from build123d import *

# Parameters (mm, degrees)
SKETCH1_R                      = 20.32
CYLINDER_DEPTH                 = 26.162
SKETCH18_R                     = 12.7
CUT_EXTRUDE10_DEPTH            = 23.368
SKETCH19_R                     = 1.905
CUT_EXTRUDE12_REACH            = 40.862
SKETCH21_R                     = 1.27
CIRPATTERN4_COUNT              = 6
CUT_EXTRUDE13_REACH            = 39.039
SKETCH22_R                     = 8.001
CUT_EXTRUDE15_REACH            = 54.431
CUT_EXTRUDE15_END_MAJOR_RADIUS = 12.573
CUT_EXTRUDE15_END_MINOR_RADIUS = 1.905
SKETCH25_R                     = 1.905
CIRPATTERN6_COUNT              = 2
SKETCH26_R                     = 1.905
CUT_EXTRUDE16_DEPTH            = 53.430547027
CUT_EXTRUDE17_DEPTH            = 39.862000188
CUT_EXTRUDE17_DEPTH_BACK       = 39.862000188
SKETCH27_W                     = 40.64
SKETCH27_H                     = 2.54


with BuildPart() as part:
    # Sketch1 → Cylinder (new body)
    with BuildSketch(Plane(origin=(0, 0, 0), x_dir=(1, 0, 0), z_dir=(0, 1, 0))):
        with Locations(Location((0, 0, 0), (0, 0, 270))):
            Circle(SKETCH1_R)
    extrude(amount=CYLINDER_DEPTH)

    # Sketch18 → Cut-Extrude10 (cut)
    with BuildSketch(Plane(origin=(0, 26.162, 0), x_dir=(1, 0, 0), z_dir=(0, 1, 0))):
        with Locations(Location((0, 0, 0), (0, 0, 270))):
            Circle(SKETCH18_R)
    extrude(amount=-CUT_EXTRUDE10_DEPTH, mode=Mode.SUBTRACT)

    # Sketch19 → Cut-Revolve7 (revolve, cut)
    with BuildSketch(Plane.XY, mode=Mode.PRIVATE) as cut_revolve7_sk:
        with Locations((12.573, 0)):
            Circle(SKETCH19_R)
    revolve(cut_revolve7_sk.sketch.rotate(Axis((0, 13.335, 0), (0, -1, 0)), 90), axis=Axis((0, 13.335, 0), (0, -1, 0)), mode=Mode.SUBTRACT)

    # Sketch21 → Cut-Extrude12 (cut, up to next)
    with BuildSketch(Plane(origin=(0, 26.162, 0), x_dir=(1, 0, 0), z_dir=(0, 1, 0)), mode=Mode.PRIVATE) as cut_extrude12_sk1:
        with Locations(Location((0, 17.78, 0), (0, 0, 270))):
            Circle(SKETCH21_R)
    cut_extrude12_tool1 = extrude(cut_extrude12_sk1.sketch, amount=-CUT_EXTRUDE12_REACH, mode=Mode.PRIVATE) & part.part
    cut_extrude12 = cut_extrude12_tool1.solids().sort_by_distance((0, 26.162, -17.78))[0]
    add(cut_extrude12, mode=Mode.SUBTRACT)

    # CirPattern4: Cut-Extrude12 ×6 about axis
    cirpattern4_axis = Axis((0, 0, 0), (0, 1, 0))
    for i in range(1, CIRPATTERN4_COUNT):
        add(cut_extrude12.rotate(cirpattern4_axis, i * 360 / CIRPATTERN4_COUNT), mode=Mode.SUBTRACT)

    # Sketch22 → Cut-Extrude13 (cut, up to next)
    with BuildSketch(Plane(origin=(0, 2.794, 0), x_dir=(1, 0, 0), z_dir=(0, 1, 0)), mode=Mode.PRIVATE) as cut_extrude13_sk1:
        with Locations(Location((0, 0, 0), (0, 0, 270))):
            Circle(SKETCH22_R)
    cut_extrude13_tool1 = extrude(cut_extrude13_sk1.sketch, amount=-CUT_EXTRUDE13_REACH, mode=Mode.PRIVATE) & part.part
    add(cut_extrude13_tool1.solids().sort_by_distance((0, 2.794, 0))[0], mode=Mode.SUBTRACT)

    # Cut-Extrude15: up to this torus (the profile starts outside it)
    cut_extrude15_end = Plane(origin=(0, 0, 0), z_dir=(0, 1, 0)) * Torus(CUT_EXTRUDE15_END_MAJOR_RADIUS, CUT_EXTRUDE15_END_MINOR_RADIUS, mode=Mode.PRIVATE)
    # Sketch25 → Cut-Extrude15 (cut, up to the surface)
    with BuildSketch(Plane(origin=(20.32, 0, 0), x_dir=(0, 0, -1), z_dir=(1, 0, 0)), mode=Mode.PRIVATE) as cut_extrude15_sk1:
        Circle(SKETCH25_R)
    cut_extrude15_tool1 = extrude(cut_extrude15_sk1.sketch, amount=-CUT_EXTRUDE15_REACH, mode=Mode.PRIVATE) - cut_extrude15_end
    cut_extrude15 = cut_extrude15_tool1.solids().sort_by_distance((20.32, 0, 0))[0]
    add(cut_extrude15, mode=Mode.SUBTRACT)

    # CirPattern6: Cut-Extrude15 ×2 about axis
    cirpattern6_axis = Axis((0, 13.335, 0), (0, -1, 0))
    for i in range(1, CIRPATTERN6_COUNT):
        add(cut_extrude15.rotate(cirpattern6_axis, i * 360 / CIRPATTERN6_COUNT), mode=Mode.SUBTRACT)

    # Sketch26 → Cut-Extrude16 (cut, through all)
    with BuildSketch(Plane(origin=(20.32, 0, 0), x_dir=(0, 0, -1), z_dir=(1, 0, 0))):
        with Locations((0, 10.922)):
            Circle(SKETCH26_R)
    extrude(amount=-CUT_EXTRUDE16_DEPTH, mode=Mode.SUBTRACT)

    # Sketch27 → Cut-Extrude17 (cut, two sides: drawn at the far end of the back side and taken through both)
    with BuildSketch(Plane.XY.offset(-CUT_EXTRUDE17_DEPTH_BACK)):
        with Locations((0, 24.892)):
            Rectangle(SKETCH27_W, SKETCH27_H)
    extrude(amount=CUT_EXTRUDE17_DEPTH + CUT_EXTRUDE17_DEPTH_BACK, mode=Mode.SUBTRACT)


solid = part.part
Source: CAD feature listing. Evaluate the final solid. Frame: model axes, mm. A direction names the side the tool comes from. Round coordinates to 2 decimals unless told otherwise and drop trailing zeros. Order: outer loops, then holes, each group sorted by start corner. A loop starts at its lowest first (then second) coordinate and runs counter-clockwise, first axis right, second up. Notation, with made-up numbers: (49, 4.5) - (89, 4.5) arc R22 cw to (89, 29.5) - close; hole circle Ø9 at (-23.5, 15). An arc over 180 degrees is marked (long way). Use a Markdown table: item, result. Add a question column.
1. Section query C-C (y = 11.5). Return the cut outline in (x, z) (3 decimals), then the cut area to 3 significant figures.
2. First-contact query: pin 1 (10 mm diameter, centred on y = 2.5, z = -13, fed in from +X); pin 2 (2.5 mm diameter, centred on y = 10.922, z = 0, fed in from -X); pin 3 (3 mm diameter, centred on x = -16, y = 7, fed in from +Z); pin 4 (1.5 mm diameter, centred on x = 7, y = 6.5, fed in from +Z). Flat tips, straight axial feed; report the tip coordinate or a pass-through.
3. Set-up query: faces 4 (the cylindrical face through (17.362, 1.905, -0.042)), 5 (the cylindrical face through (-12.4, 13.35, -2.75)), 6 (the cylindrical face through (-17.362, 1.905, 0.042)), 7 (the cylindrical face through (-16.47, 11.98, -9.57)). Return all of +Z, -Z, +X, -X, +Y, -Y with unobstructed straight access to the full face (end or side cutting, diameter ignored); none if empty.
4. Section query A-A (z = 0). Return the cut outline in (x, y) (3 decimals), then the cut area to 3 significant figures.
5. Section query D-D (x = -15). Return the cut outline in (y, z) (3 decimals), then the cut area to 3 significant figures.
6. Mould query, pull axis Z, two halves, no side actions, for faces 1 (the flat face through (8, 0, 2)), 2 (the cylindrical face through (14.54, 11.976, -7.954)), 3 (the cylindrical face through (20.147, 11.646, -2.645)). Classes: +Z half, -Z half, draft (parallel to the pull), parting line (faces both ways), or undercut.
7. Line query: probe 1 along Z at (x, y) = (16.5, 21.75); probe 2 along X at (y, z) = (13.25, 8.89); probe 3 along Z at (x, y) = (7, 8.5). Output: solid intervals per line, ascending.
8. Section query B-B (x = 0). Return the cut outline in (y, z) (3 decimals), then the cut area to 3 significant figures.
Derived:
| question | item | result |
|---|---|---|
| 1 | outline | (-20.239, -1.815) arc R20.32 ccw to (20.239, -1.815) - (12.57, -1.815) arc R12.7 cw to (-12.57, -1.815) - close; (-20.239, 1.815) - (-12.57, 1.815) arc R12.7 cw to (12.57, 1.815) - (20.239, 1.815) arc R20.32 ccw to start; hole circle Ø2.54 at (-15.398, -8.89); hole circle Ø2.54 at (-15.398, 8.89); hole circle Ø2.54 at (0, -17.78); hole circle Ø2.54 at (0, 17.78); hole circle Ø2.54 at (15.398, -8.89); hole circle Ø2.54 at (15.398, 8.89) |
| 1 | area | 705 mm2 |
| 2 | pin 1 | x = 18.68 |
| 2 | pin 2 | through |
| 2 | pin 3 | z = 14.24 |
| 2 | pin 4 | z = 19.33 |
| 3 | face 4 | +X, -Y |
| 3 | face 5 | +Y |
| 3 | face 6 | -X, -Y |
| 3 | face 7 | +Y, -Y |
| 4 | outline | (-20.32, 1.905) - (-12.573, 1.905) arc R1.905 cw to (-10.668, 0) - (-8.001, 0) - (-8.001, 2.794) - (-12.7, 2.794) - (-12.7, 9.017) - (-20.32, 9.017) - close; (-20.32, 12.827) - (-12.7, 12.827) - (-12.7, 23.622) - (-20.32, 23.622) - close; (8.001, 0) - (10.668, 0) arc R1.905 cw to (12.573, 1.905) - (20.32, 1.905) - (20.32, 9.017) - (12.7, 9.017) - (12.7, 2.794) - (8.001, 2.794) - close; (12.7, 12.827) - (20.32, 12.827) - (20.32, 23.622) - (12.7, 23.622) - close |
| 4 | area | 293 mm2 |
| 5 | outline | (0, -13.708) - (23.622, -13.708) - (23.622, -10.096) - (0, -10.096) - close; (0, -7.684) - (23.622, -7.684) - (23.622, 7.684) - (0, 7.684) - (0, 1.905) arc R1.905 cw to (0, -1.905) - close; (0, 10.096) - (23.622, 10.096) - (23.622, 13.708) - (0, 13.708) - close; hole circle Ø3.81 at (10.922, 0) |
| 5 | area | 517 mm2 |
| 6 | face 1 | draft |
| 6 | face 2 | undercut |
| 6 | face 3 | parting line |
| 7 | probe 1 | -11.86 to -9.52, -8.26 to 8.26, 9.52 to 11.86 |
| 7 | probe 2 | -18.27 to -16.67, -14.13 to -9.07, 9.07 to 14.13, 16.67 to 18.27 |
| 7 | probe 3 | -19.08 to -10.6, 10.6 to 19.08 |
| 8 | outline | (0, -20.32) - (23.622, -20.32) - (23.622, -19.05) - (0, -19.05) - close; (0, -16.51) - (23.622, -16.51) - (23.622, -12.7) - (2.794, -12.7) - (2.794, -8.001) - (0, -8.001) - (0, -10.668) arc R1.905 cw to (0, -14.478) - close; (0, 8.001) - (2.794, 8.001) - (2.794, 12.7) - (23.622, 12.7) - (23.622, 16.51) - (0, 16.51) - (0, 14.478) arc R1.905 cw to (0, 10.668) - close; (0, 19.05) - (23.622, 19.05) - (23.622, 20.32) - (0, 20.32) - close |
| 8 | area | 255 mm2 |
